```python
from build123d import *

# Parameters (mm, degrees)
SKETCH1_6_R         = 28.2
SKETCH1_6_R_2       = 3
BOSS_EXTRUDE4_DEPTH = 10
FILLET4_R           = 1.5


with BuildPart() as part:
    # Sketch1_6 → Boss-Extrude4 (new body)
    with BuildSketch(Plane.XY):
        Circle(SKETCH1_6_R)
        with BuildLine():
            ThreePointArc((5.866209712, 8.098616155), (3.505253449, 9.36553246), (0.892648331, 9.960079265))
            Line((0.892648331, 9.960079265), (2.101110424, 23.44397635))
            ThreePointArc((2.101110424, 23.44397635), (2.670485373, 24.491199978), (3.823764506, 24.792550937))
            ThreePointArc((3.823764506, 24.792550937), (8.793169539, 23.494082796), (13.393949598, 21.210701807))
            ThreePointArc((13.393949598, 21.210701807), (14.065968099, 20.226193659), (13.807850128, 19.062475363))
            Line((13.807850128, 19.062475363), (5.866209712, 8.098616155))
        make_face(mode=Mode.SUBTRACT)
        with BuildLine():
            ThreePointArc((-9.946712181, 1.030978557), (-9.863415755, -1.647127697), (-9.072005832, -4.206983501))
            Line((-9.072005832, -4.206983501), (-21.353634297, -9.902373172))
            ThreePointArc((-21.353634297, -9.902373172), (-22.545244036, -9.932891816), (-23.382861189, -9.084798269))
            ThreePointArc((-23.382861189, -9.084798269), (-24.74305731, -4.131933198), (-25.065981396, 0.994149706))
            ThreePointArc((-25.065981396, 0.994149706), (-24.54938158, 2.068388873), (-23.412512987, 2.426711301))
            Line((-23.412512987, 2.426711301), (-9.946712181, 1.030978557))
        make_face(mode=Mode.SUBTRACT)
        with BuildLine():
            ThreePointArc((-5.866209712, -8.098616155), (-3.505253449, -9.36553246), (-0.892648331, -9.960079265))
            Line((-0.892648331, -9.960079265), (-2.101110424, -23.44397635))
            ThreePointArc((-2.101110424, -23.44397635), (-2.670485373, -24.491199978), (-3.823764506, -24.792550937))
            ThreePointArc((-3.823764506, -24.792550937), (-8.793169539, -23.494082796), (-13.393949598, -21.210701807))
            ThreePointArc((-13.393949598, -21.210701807), (-14.065968099, -20.226193659), (-13.807850128, -19.062475363))
            Line((-13.807850128, -19.062475363), (-5.866209712, -8.098616155))
        make_face(mode=Mode.SUBTRACT)
        with BuildLine():
            ThreePointArc((9.946712181, -1.030978557), (9.863415755, 1.647127697), (9.072005832, 4.206983501))
            Line((9.072005832, 4.206983501), (21.353634297, 9.902373172))
            ThreePointArc((21.353634297, 9.902373172), (22.545244036, 9.932891816), (23.382861189, 9.084798269))
            ThreePointArc((23.382861189, 9.084798269), (24.74305731, 4.131933198), (25.065981396, -0.994149706))
            ThreePointArc((25.065981396, -0.994149706), (24.54938158, -2.068388873), (23.412512987, -2.426711301))
            Line((23.412512987, -2.426711301), (9.946712181, -1.030978557))
        make_face(mode=Mode.SUBTRACT)
        with Locations((-18.369803336, -15.132426289)):
            Circle(SKETCH1_6_R_2, mode=Mode.SUBTRACT)
        with Locations((3.920163919, -23.474929496)):
            Circle(SKETCH1_6_R_2, mode=Mode.SUBTRACT)
        with Locations((22.289967255, -8.342503208)):
            Circle(SKETCH1_6_R_2, mode=Mode.SUBTRACT)
        with Locations((-22.289967255, 8.342503208)):
            Circle(SKETCH1_6_R_2, mode=Mode.SUBTRACT)
        with Locations((18.369803336, 15.132426289)):
            Circle(SKETCH1_6_R_2, mode=Mode.SUBTRACT)
        with Locations((-3.920163919, 23.474929496)):
            Circle(SKETCH1_6_R_2, mode=Mode.SUBTRACT)
        with BuildLine():
            ThreePointArc((-0.15563191, 3.046026708), (1.939239503, -2.354113453), (-2.95986762, 0.735991626))
            Line((-2.95986762, 0.735991626), (-0.15563191, 3.046026708))
        make_face(mode=Mode.SUBTRACT)
    extrude(amount=-BOSS_EXTRUDE4_DEPTH)

    # Fillet4
    fillet4_edges = [part.edges().sort_by_distance(p)[0] for p in [
        (-5.866209712, -8.098616155, -5),
        (-0.892648331, -9.960079265, -5),
        (9.072005832, 4.206983501, -5),
        (9.946712181, -1.030978557, -5),
        (0.892648331, 9.960079265, -5),
        (5.866209712, 8.098616155, -5),
        (-9.072005832, -4.206983501, -5),
        (-9.946712181, 1.030978557, -5),
    ]]
    fillet(fillet4_edges, radius=FILLET4_R)


solid = part.part
```
Source: CAD feature listing. Evaluate the final solid. Frame: model axes, mm. Round coordinates to 2 decimals unless told otherwise and drop trailing zeros. Loops run counter-clockwise (first coordinate to the right, second up) from the corner with the lowest first, then second, coordinate; pieces in that order, holes last.
(1) Contact query for flat-ended pins moving along their axis: pin 1 Ø9.5 at (x, y) = (-3.92, 23.47) entering from -Z; pin 2 Ø5 at (x, z) = (10.5, -1.5) entering from +Y; pin 3 Ø2 at (y, z) = (21.5, -8) entering from -X; pin 4 Ø2 at (x, z) = (8.5, -6) entering from -Y. Output: stop coordinate, or through.
From the geometry:
pin 1: stops at z = -10
pin 2: stops at y = 27.04
pin 3: stops at x = -19.36
pin 4: stops at y = -27.18
(2) Material intervals for probe 1 along X at (y, z) = (15, -7.25); probe 2 along Y at (x, z) = (22.5, -4.25); probe 3 along Y at (x, z) = (6.5, -2), sorted ascending.
From the geometry:
probe 1: x = -23.88 to 1.34, 10.87 to 15.37, 21.37 to 23.88
probe 2: y = -17 to -11.34, -5.35 to -2.33, 9.95 to 17
probe 3: y = -27.44 to -25.01, -21.94 to 9.02, 24.23 to 27.44
(3) Section query C-C (z = -1). Give the number of separate pieces and of enclosed holes in the cut face, and give its area (3 significant figures).
From the geometry:
separate pieces: 1
enclosed holes: 11
area: 1,740 mm2
(4) Pull-direction query (X, two-part tool) for faces 1 (the flat face through (1.552, 17.315, -4.93)), 2 (the flat face through (0, -6, -10)); classes: +X half, -X half, draft (parallel to the pull), parting line (faces both ways), or undercut.
From the geometry:
face 1: undercut
face 2: draft
(5) Section query B-B (y = -7.5). Output: boundary loops of the cut face in (x, z).
From the geometry:
outline: (-27.18, -10) - (-23.94, -10) - (-23.94, 0) - (-27.18, 0) - close; (-16.17, -10) - (19.41, -10) - (19.41, 0) - (-16.17, 0) - close; (25.17, -10) - (27.18, -10) - (27.18, 0) - (25.17, 0) - close
(6) Section query A-A (y = -14). Output: boundary loops of the cut face in (x, z), and give its area (3 significant figures).
From the geometry:
outline: (-24.48, -10) - (-21.15, -10) - (-21.15, 0) - (-24.48, 0) - close; (-15.59, -10) - (-10.14, -10) - (-10.14, 0) - (-15.59, 0) - close; (-1.25, -10) - (24.48, -10) - (24.48, 0) - (-1.25, 0) - close
area: 345 mm2
